```python
from build123d import *

# Parameters (mm, degrees)
SKETCH1_R           = 14
BOSS_EXTRUDE1_DEPTH = 16
CUT_EXTRUDE1_REACH  = 27.456
SKETCH2_R           = 9
CUT_EXTRUDE2_DEPTH  = 26.455844123
BOSS_EXTRUDE2_START = 11
SKETCH4_R           = 5
BOSS_EXTRUDE2_DEPTH = 3
BOSS_EXTRUDE2_DRAFT = -45
SKETCH5_R           = 8
BOSS_EXTRUDE3_DEPTH = 5
SKETCH6_R           = 5
CUT_EXTRUDE3_DEPTH  = 4
CUT_EXTRUDE4_START  = 17
SKETCH7_R           = 1.5
CUT_EXTRUDE4_DEPTH  = 5
FILLET1_R           = 1


with BuildPart() as part:
    # Sketch1 → Boss-Extrude1 (new body)
    with BuildSketch(Plane.XY):
        Circle(SKETCH1_R)
    extrude(amount=BOSS_EXTRUDE1_DEPTH)

    # Sketch2 → Cut-Extrude1 (cut, up to next)
    with BuildSketch(Plane.XY.offset(16), mode=Mode.PRIVATE) as cut_extrude1_sk1:
        Circle(SKETCH2_R)
    cut_extrude1_tool1 = extrude(cut_extrude1_sk1.sketch, amount=-CUT_EXTRUDE1_REACH, mode=Mode.PRIVATE) & part.part
    add(cut_extrude1_tool1.solids().sort_by_distance((0, 0, 16))[0], mode=Mode.SUBTRACT)

    # Sketch3 → Cut-Extrude2 (cut, through all)
    with BuildSketch(Plane.XY.offset(16)):
        Polygon((-14, -5.5), (14, -5), (14, -14), (-14, -14), align=None)
    extrude(amount=-CUT_EXTRUDE2_DEPTH, mode=Mode.SUBTRACT)


with BuildPart() as boss_extrude2_tool:
    # Sketch4 → Boss-Extrude2 (with draft: the straight prism first)
    with BuildSketch(Plane(origin=(0, 0, 0), x_dir=(-1, 0, 0), z_dir=(0, 1, 0)).offset(BOSS_EXTRUDE2_START)):
        with Locations((0, 8)):
            Circle(SKETCH4_R)
    extrude(amount=BOSS_EXTRUDE2_DEPTH)
    # Boss-Extrude2: the draft: its side faces are tilted about the plane it starts from
    boss_extrude2_sides = [boss_extrude2_tool.faces().sort_by_distance(p)[0] for p in [
        (5, 12.5, 8),
    ]]
    draft(boss_extrude2_sides, Plane(origin=(0, 0, 0), x_dir=(-1, 0, 0), z_dir=(0, 1, 0)).offset(BOSS_EXTRUDE2_START), BOSS_EXTRUDE2_DRAFT)


with BuildPart() as part_1:
    add(part.part)

    # Boss-Extrude2: add boss_extrude2_tool
    add(boss_extrude2_tool.part)

    # Sketch5 → Boss-Extrude3 (add)
    with BuildSketch(Plane(origin=(0, 14, 0), x_dir=(1, 0, 0), z_dir=(0, 1, 0))):
        with Locations(Location((0, -8, 0), (0, 0, 270))):
            Circle(SKETCH5_R)
    extrude(amount=BOSS_EXTRUDE3_DEPTH)

    # Sketch6 → Cut-Extrude3 (cut)
    with BuildSketch(Plane(origin=(0, 19, 0), x_dir=(1, 0, 0), z_dir=(0, 1, 0))):
        with Locations(Location((0, -8, 0), (0, 0, 270))):
            Circle(SKETCH6_R)
    extrude(amount=-CUT_EXTRUDE3_DEPTH, mode=Mode.SUBTRACT)

    # Sketch7 → Cut-Extrude4 (cut)
    with BuildSketch(Plane.XY.offset(CUT_EXTRUDE4_START)):
        with Locations(Location((0, 16.5, 0), (0, 0, 270))):
            Circle(SKETCH7_R)
    extrude(amount=-CUT_EXTRUDE4_DEPTH, mode=Mode.SUBTRACT)

    # Fillet1
    fillet1_edges = [part_1.edges().sort_by_distance(p)[0] for p in [
        (7.403251486, -5.117799081, 8),
        (-7.215811257, -5.378853772, 8),
    ]]
    fillet(fillet1_edges, radius=FILLET1_R)


solid = part_1.part
```
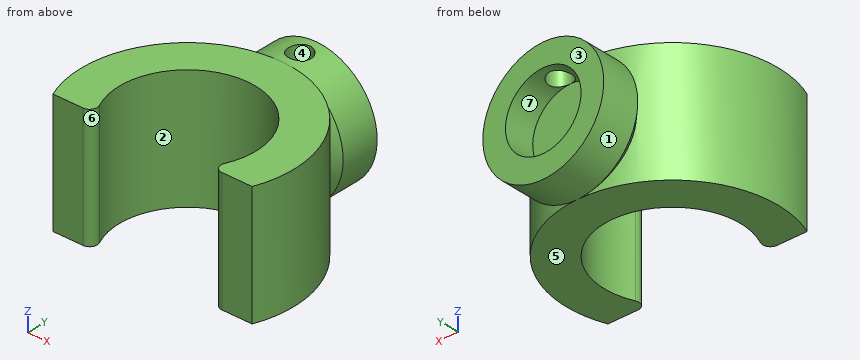
Can you work these out from the model? Positions are in its coordinate system, mm. Face numbers are marked on the shaded views. A direction names the side the tool comes from. Give positions to 0.01 mm unless a question says otherwise; leave off trailing zeros. Loops run counter-clockwise (first coordinate to the right, second up) from the corner with the lowest first, then second, coordinate; pieces in that order, holes last. Notation, with made-up numbers: M -5.75,-10.5 L 10.25,-10.5 A17 ccw 10.25,16.5 Z; hole C 80,83.25 d5. An arc over 180 degrees is marked long. Use CSV: the item, a comma, the result in double quotes. Start each with the question number.
1. Imagine slicing it at A-A, the plane y = -2.5. Write out the boundary of the cut face in (x, z).
2. If I drill on L1, parallel to X at y = 17.55, z = 8; L2, parallel to Y at x = 0, z = 13.75; L3, parallel to X at y = 0, z = 3.5, over which ranges is the centre line in solid material (lowest first)?
3. Imagine slicing it at B-B, the plane z = 8. Write out the boundary of the cut face in (x, y).
4. For P1, Ø1.5, axis at y = 5, z = 7.5, coming from the +X side; P2, Ø1.5, axis at y = 2.5, z = 14, coming from the -X side; P3, Ø4, axis at x = 8, y = -2.5, coming from the -Z side; P4, Ø3, axis at x = -7.5, z = 9.5, coming from the -Y side, each with a flat end and sliding along its axis, tell me the tip position at first contact or that it passes through.
5. If we mould it in two halves opening along X, with no side actions, what happens to the marked faces 1, 2 and 3? For each: released by +X, released by -X, zero draft, split by the parting line, or undercut.
6. On a 3-axis mill with a long thin cutter (end or side, diameter ignored), from which of +Z, -Z, +X, -X, +Y, -Y can I reach the whole of each face in a straight line? I mean the marked faces 4, 5, 6 and 7. Say none if no direction works.
7. Imagine slicing it at D-D, the plane y = 15.75. Write out the boundary of the cut face in (x, z), plus the area to 3 significant figures.
8. Imagine slicing it at C-C, the plane y = 0.5. Write out the boundary of the cut face in (x, z), plus the area to 3 significant figures.
Response values:
1,outline,"M -13.77,0 L -8.65,0 L -8.65,16 L -13.77,16 Z; M 8.65,0 L 13.77,0 L 13.77,16 L 8.65,16 Z"
2,L1,"-8 to -5, 5 to 8"
2,L2,"9 to 15, 18 to 19"
2,L3,"-14 to -9, 9 to 14"
3,outline,"M -12.88,-5.48 L -8.96,-5.41 A1 ccw -8.08,-3.97 A9 cw long 8.21,-3.68 A1 ccw 9.14,-5.09 L 13.07,-5.02 A14 ccw 6.43,12.43 L 8,14 L 8,19 L 5,19 L 5,15 L -5,15 L -5,19 L -8,19 L -8,14 L -6.43,12.43 A14 ccw Z"
4,P1,"x = 13.34"
4,P2,"x = -13.89"
4,P3,"z = 0"
4,P4,"y = -5.41"
5,face 1,"split by the parting line"
5,face 2,"undercut"
5,face 3,"zero draft"
6,face 4,"+Z"
6,face 5,"-Z, +X, -X, +Y, -Y"
6,face 6,"+Z, -Z"
6,face 7,"+Y"
7,outline,"M -1.3,12.83 L -1.3,15.89 A8 ccw long 1.3,15.89 L 1.3,12.83 A5 cw long Z"
7,area,"115 mm^2"
8,outline,"M -13.99,0 L -8.99,0 L -8.99,16 L -13.99,16 Z; M 8.99,0 L 13.99,0 L 13.99,16 L 8.99,16 Z"
8,area,"160 mm^2"
